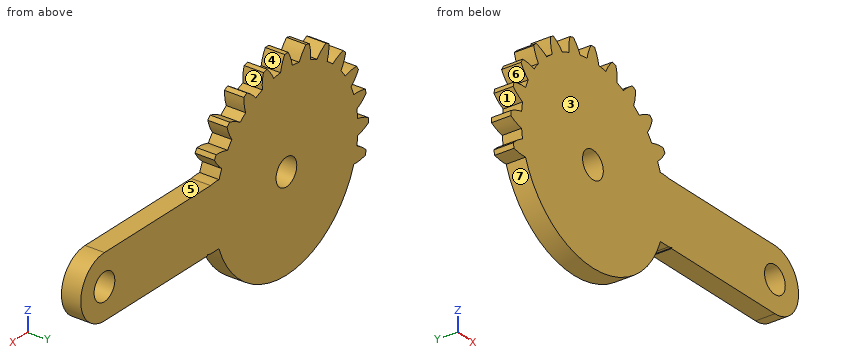
```python
from build123d import *

# Parameters (mm, degrees)
SKETCH_1_R      = 7
EXTRUDE_2_DEPTH = 10


with BuildPart() as part:
    # 草图1 → 凸台-拉伸2 (new body)
    with BuildSketch(Plane(origin=(0, 0, 0), x_dir=(1, 0, 0), z_dir=(0, 1, 0))):
        with BuildLine():
            Line((51.235128203, 16), (45.636494169, 16))
            ThreePointArc((45.636494169, 16), (0.158881993, 48.359739004), (-45.530376716, 16.299521346))
            ThreePointArc((-45.530376716, 16.299521346), (-49.445367881, 16.258078448), (-53.288564328, 15.510606432))
            ThreePointArc((-53.288564328, 15.510606432), (-53.608883359, 14.364457003), (-53.904553655, 13.211702966))
            ThreePointArc((-53.904553655, 13.211702966), (-50.949983909, 10.642774988), (-47.580223553, 8.649388802))
            ThreePointArc((-47.580223553, 8.649388802), (-47.946273496, 6.312246656), (-48.197593301, 3.96))
            ThreePointArc((-48.197593301, 3.96), (-51.968458166, 2.906694959), (-55.487240876, 1.19))
            ThreePointArc((-55.487240876, 1.19), (-55.5, 0), (-55.487240876, -1.19))
            ThreePointArc((-55.487240876, -1.19), (-51.968458166, -2.906694959), (-48.197593301, -3.96))
            ThreePointArc((-48.197593301, -3.96), (-47.946273496, -6.312246656), (-47.580223553, -8.649388802))
            ThreePointArc((-47.580223553, -8.649388802), (-50.949983909, -10.642774988), (-53.904553655, -13.211702966))
            ThreePointArc((-53.904553655, -13.211702966), (-53.608883359, -14.364457003), (-53.288564328, -15.510606432))
            ThreePointArc((-53.288564328, -15.510606432), (-49.445367881, -16.258078448), (-45.530376716, -16.299521346))
            ThreePointArc((-45.530376716, -16.299521346), (-44.678814192, -18.506570789), (-43.7203402, -20.669336051))
            ThreePointArc((-43.7203402, -20.669336051), (-46.459352447, -23.466957407), (-48.648360184, -26.713050207))
            ThreePointArc((-48.648360184, -26.713050207), (-48.06440991, -27.75), (-47.458360184, -28.774190668))
            ThreePointArc((-47.458360184, -28.774190668), (-43.552657488, -28.501500759), (-39.7603402, -27.528257249))
            ThreePointArc((-39.7603402, -27.528257249), (-38.366567536, -29.439702707), (-36.880987913, -31.280702206))
            ThreePointArc((-36.880987913, -31.280702206), (-38.802592894, -34.691905461), (-40.076861362, -38.393947223))
            ThreePointArc((-40.076861362, -38.393947223), (-39.244426356, -39.244426356), (-38.393947223, -40.076861362))
            ThreePointArc((-38.393947223, -40.076861362), (-34.691905461, -38.802592894), (-31.280702206, -36.880987913))
            ThreePointArc((-31.280702206, -36.880987913), (-29.439702707, -38.366567536), (-27.528257249, -39.7603402))
            ThreePointArc((-27.528257249, -39.7603402), (-28.501500759, -43.552657488), (-28.774190668, -47.458360184))
            ThreePointArc((-28.774190668, -47.458360184), (-27.75, -48.06440991), (-26.713050207, -48.648360184))
            ThreePointArc((-26.713050207, -48.648360184), (-23.466957407, -46.459352447), (-20.669336051, -43.7203402))
            ThreePointArc((-20.669336051, -43.7203402), (-18.506570789, -44.678814192), (-16.299521346, -45.530376716))
            ThreePointArc((-16.299521346, -45.530376716), (-16.258078448, -49.445367881), (-15.510606432, -53.288564328))
            ThreePointArc((-15.510606432, -53.288564328), (-14.364457003, -53.608883359), (-13.211702966, -53.904553655))
            ThreePointArc((-13.211702966, -53.904553655), (-10.642774988, -50.949983909), (-8.649388802, -47.580223553))
            ThreePointArc((-8.649388802, -47.580223553), (-6.312246656, -47.946273496), (-3.96, -48.197593301))
            ThreePointArc((-3.96, -48.197593301), (-2.906694959, -51.968458166), (-1.19, -55.487240876))
            ThreePointArc((-1.19, -55.487240876), (0, -55.5), (1.19, -55.487240876))
            ThreePointArc((1.19, -55.487240876), (2.906694959, -51.968458166), (3.96, -48.197593301))
            ThreePointArc((3.96, -48.197593301), (6.312246656, -47.946273496), (8.649388802, -47.580223553))
            ThreePointArc((8.649388802, -47.580223553), (10.642774988, -50.949983909), (13.211702966, -53.904553655))
            ThreePointArc((13.211702966, -53.904553655), (14.364457003, -53.608883359), (15.510606432, -53.288564328))
            ThreePointArc((15.510606432, -53.288564328), (16.258078448, -49.445367881), (16.299521346, -45.530376716))
            ThreePointArc((16.299521346, -45.530376716), (18.506570789, -44.678814192), (20.669336051, -43.7203402))
            ThreePointArc((20.669336051, -43.7203402), (23.466957407, -46.459352447), (26.713050207, -48.648360184))
            ThreePointArc((26.713050207, -48.648360184), (27.75, -48.06440991), (28.774190668, -47.458360184))
            ThreePointArc((28.774190668, -47.458360184), (28.501500759, -43.552657488), (27.528257249, -39.7603402))
            ThreePointArc((27.528257249, -39.7603402), (29.439702707, -38.366567536), (31.280702206, -36.880987913))
            ThreePointArc((31.280702206, -36.880987913), (34.691905461, -38.802592894), (38.393947223, -40.076861362))
            ThreePointArc((38.393947223, -40.076861362), (39.244426356, -39.244426356), (40.076861362, -38.393947223))
            ThreePointArc((40.076861362, -38.393947223), (38.802592894, -34.691905461), (36.880987913, -31.280702206))
            ThreePointArc((36.880987913, -31.280702206), (38.366567536, -29.439702707), (39.7603402, -27.528257249))
            ThreePointArc((39.7603402, -27.528257249), (43.552657488, -28.501500759), (47.458360184, -28.774190668))
            ThreePointArc((47.458360184, -28.774190668), (48.06440991, -27.75), (48.648360184, -26.713050207))
            ThreePointArc((48.648360184, -26.713050207), (46.459352447, -23.466957407), (43.7203402, -20.669336051))
            ThreePointArc((43.7203402, -20.669336051), (44.678814192, -18.506570789), (45.530376716, -16.299521346))
            ThreePointArc((45.530376716, -16.299521346), (48.39269803, -16.339186258), (51.235128203, -16))
            Line((51.235128203, -16), (123, -16))
            ThreePointArc((123, -16), (139, 0), (123, 16))
            Line((123, 16), (53.143673189, 16))
            ThreePointArc((53.143673189, 16), (53.216681334, 15.755469774), (53.288564328, 15.510606432))
            ThreePointArc((53.288564328, 15.510606432), (52.267828339, 15.780403272), (51.235128203, 16))
        make_face()
        with Locations(Location((0, 0, 0), (0, 0, 270))):
            Circle(SKETCH_1_R, mode=Mode.SUBTRACT)
        with Locations(Location((123, 0, 0), (0, 0, 270))):
            Circle(SKETCH_1_R, mode=Mode.SUBTRACT)
    extrude(amount=EXTRUDE_2_DEPTH)


solid = part.part
```
Build history of the part. All positions in model axes, mm. Face numbers are marked on the shaded views. A direction names the side the tool comes from. Coordinates: 2 decimals unless noted, no trailing zeros. Order: outer loops, then holes, each group sorted by start corner. A loop starts at its lowest first (then second) coordinate and runs counter-clockwise, first axis right, second up. Notation, with made-up numbers: (50, -15) -> (105, -15) arc R17 ccw to (105, 4) -> close; hole circle Ø5 at (34.5, 73.5). An arc over 180 degrees is marked (long way). Answer in a Markdown table with one row per item. Add a question column.
Q1. Wall check: line 1 along X through (y, z) = (2, 0); line 2 along Z through (x, y) = (85.5, 5.25); line 3 along X through (y, z) = (6.75, 46). Give the ranges that are in metal, low to high. Write a range as [from, to].
Q2. Band-saw the part on C-C, the plane z = -37. List the corners of the cut face in (x, y), then the cut area to 3 significant figures.
Q3. Band-saw the part on A-A, the plane y = 5.5. Give the number of separate pieces and of enclosed holes in the cut face, then the cut area to 3 significant figures.
Q4. Which spindle directions (+Z, -Z, +X, -X, +Y, -Y) get a long thin tool onto all of the face, cutting with end or side? Do the marked faces 1, 2, 3 and 4. Say none if no direction does.
Q5. Drop flat-ended pins along their axis: pin 1 (4 mm diameter, centred on y = 7, z = 35, fed in from -X); pin 2 (5 mm diameter, centred on y = 4.5, z = 22, fed in from +X); pin 3 (1.7 mm diameter, centred on x = 48.5, y = 4, fed in from -Z); pin 4 (8.5 mm diameter, centred on x = 123, z = 0, fed in from +Y). Give the stop position or say it passes through.
Q6. Mould opens along Z. For the marked faces 5, 6 and 7 say: +Z half, -Z half, draft (parallel to the pull), parting line (faces both ways), or undercut.
Q7. Band-saw the part on B-B, the plane x = 97.5. List the corners of the cut face in (y, z), then the cut area to 3 significant figures.
Answers follow:
| question | item | result |
|---|---|---|
| 1 | line 1 | [-55.5, -7], [7, 116], [130, 139] |
| 1 | line 2 | [-16, 16] |
| 1 | line 3 | [-28.76, -22.92], [-16.33, 16.33], [22.92, 28.76] |
| 2 | outline | (-31.14, 0) -> (31.14, 0) -> (31.14, 10) -> (-31.14, 10) -> close |
| 2 | area | 623 mm^2 |
| 3 | separate pieces | 1 |
| 3 | enclosed holes | 2 |
| 3 | area | 10,300 mm^2 |
| 4 | face 1 | -X, +Y, -Y |
| 4 | face 2 | +Y, -Y |
| 4 | face 3 | +Z, -Z, +X, -X, -Y |
| 4 | face 4 | +Z, +Y, -Y |
| 5 | pin 1 | x = -39.68 |
| 5 | pin 2 | x = 47.25 |
| 5 | pin 3 | z = -16 |
| 5 | pin 4 | through |
| 6 | face 5 | +Z half |
| 6 | face 6 | undercut |
| 6 | face 7 | -Z half |
| 7 | outline | (0, -16) -> (10, -16) -> (10, 16) -> (0, 16) -> close |
| 7 | area | 320 mm^2 |
